```python
from build123d import *

# Parameters (mm, degrees)
SKETCH1_R           = 1.275
BOSS_EXTRUDE1_DEPTH = 6.5
SKETCH2_W           = 3.53
SKETCH2_H           = 1.96
BOSS_EXTRUDE2_DEPTH = 1.45
FILLET1_R           = 0.7
SKETCH3_W           = 3.2
SKETCH3_H           = 0.56
SKETCH3_H_2         = 0.5
BOSS_EXTRUDE3_DEPTH = 0.9
SKETCH4_W           = 1.2
SKETCH4_H           = 0.56
SKETCH4_H_2         = 0.5
BOSS_EXTRUDE4_DEPTH = 3.47
FILLET2_R           = 0.59


with BuildPart() as part:
    # Sketch1 → Boss-Extrude1 (new body)
    with BuildSketch(Plane(origin=(0, 0, 0), x_dir=(0, 0, -1), z_dir=(1, 0, 0))):
        with BuildLine():
            Line((-37.373122581, 0), (-34.673122581, 0))
            Line((-34.673122581, 0), (-34.673122581, -0.45))
            Line((-34.673122581, -0.45), (-30.873122581, -0.45))
            Line((-30.873122581, -0.45), (-30.873122581, 0))
            Line((-30.873122581, 0), (-24.973122581, 0))
            Line((-24.973122581, 0), (-24.973122581, -0.45))
            Line((-24.973122581, -0.45), (-21.173122581, -0.45))
            Line((-21.173122581, -0.45), (-21.173122581, 0))
            Line((-21.173122581, 0), (-18.673122581, 0))
            ThreePointArc((-18.673122581, 0), (-18.31956919, 0.146446609), (-18.173122581, 0.5))
            Line((-18.173122581, 0.5), (-18.173122581, 9.02))
            ThreePointArc((-18.173122581, 9.02), (-18.31956919, 9.373553391), (-18.673122581, 9.52))
            Line((-18.673122581, 9.52), (-28.173122581, 9.52))
            Line((-28.173122581, 9.52), (-28.173122581, 10.16))
            Line((-28.173122581, 10.16), (-37.373122581, 10.16))
            ThreePointArc((-37.373122581, 10.16), (-37.726675972, 10.013553391), (-37.873122581, 9.66))
            Line((-37.873122581, 9.66), (-37.873122581, 0.5))
            ThreePointArc((-37.873122581, 0.5), (-37.726675972, 0.146446609), (-37.373122581, 0))
        make_face()
        with Locations((-32.773122581, 2.525)):
            Circle(SKETCH1_R, mode=Mode.SUBTRACT)
        with Locations((-23.073122581, 2.525)):
            Circle(SKETCH1_R, mode=Mode.SUBTRACT)
    extrude(amount=BOSS_EXTRUDE1_DEPTH)

    # Sketch2 → Boss-Extrude2 (add)
    with BuildSketch(Plane(origin=(0, 10.16, 0), x_dir=(1, 0, 0), z_dir=(0, 1, 0))):
        with Locations((3.635, -30.693122581)):
            Rectangle(SKETCH2_W, SKETCH2_H)
    extrude(amount=BOSS_EXTRUDE2_DEPTH)

    # Fillet1
    fillet1_edges = [part.edges().sort_by_distance(p)[0] for p in [
        (3.635, 11.61, 31.673122581),
        (3.635, 11.61, 29.713122581),
    ]]
    fillet(fillet1_edges, radius=FILLET1_R)

    # Sketch3 → Boss-Extrude3 (add)
    with BuildSketch(Plane(origin=(0, 0, 0), x_dir=(-1, 0, 0), z_dir=(0, -1, 0))):
        with Locations((-3.25, -36.193122581)):
            Rectangle(SKETCH3_W, SKETCH3_H)
        with Locations((-3.25, -27.223122581)):
            Rectangle(SKETCH3_W, SKETCH3_H_2)
        with Locations((-3.25, -20.023122581)):
            Rectangle(SKETCH3_W, SKETCH3_H_2)
    extrude(amount=BOSS_EXTRUDE3_DEPTH)

    # Sketch4 → Boss-Extrude4 (add)
    with BuildSketch(Plane(origin=(0, -0.9, 0), x_dir=(-1, 0, 0), z_dir=(0, -1, 0))):
        with Locations((-3.25, -36.193122581)):
            Rectangle(SKETCH4_W, SKETCH4_H)
        with Locations((-3.25, -27.223122581)):
            Rectangle(SKETCH4_W, SKETCH4_H_2)
        with Locations((-3.25, -20.023122581)):
            Rectangle(SKETCH4_W, SKETCH4_H_2)
    extrude(amount=BOSS_EXTRUDE4_DEPTH)

    # Fillet2
    fillet2_edges = [part.edges().sort_by_distance(p)[0] for p in [
        (2.65, -4.37, 36.193122581),
        (3.85, -4.37, 36.193122581),
        (2.65, -4.37, 27.223122581),
        (3.85, -4.37, 27.223122581),
        (3.85, -4.37, 20.023122581),
        (2.65, -4.37, 20.023122581),
    ]]
    fillet(fillet2_edges, radius=FILLET2_R)


solid = part.part
```
Work out the finished part from the listing and answer in its coordinate system (mm). A direction names the side the tool comes from. Round coordinates to 2 decimals unless told otherwise and drop trailing zeros. Loops run counter-clockwise (first coordinate to the right, second up) from the corner with the lowest first, then second, coordinate; pieces in that order, holes last.
(1) The part is cut by section C-C, the plane x = 0.75. Give the vertices of the cut face in (y, z) (3 decimals).
Computed values:
outline: (-0.45, 21.173) - (0, 21.173) - (0, 18.673) arc R0.5 ccw to (0.5, 18.173) - (9.02, 18.173) arc R0.5 ccw to (9.52, 18.673) - (9.52, 28.173) - (10.16, 28.173) - (10.16, 37.373) arc R0.5 ccw to (9.66, 37.873) - (0.5, 37.873) arc R0.5 ccw to (0, 37.373) - (0, 34.673) - (-0.45, 34.673) - (-0.45, 30.873) - (0, 30.873) - (0, 24.973) - (-0.45, 24.973) - close; hole circle Ø2.55 at (2.525, 23.073); hole circle Ø2.55 at (2.525, 32.773)
(2) Each of these flat-tipped pins is pushed along its axis until it touches: P1, Ø1, axis at y = 4.5, z = 24, coming from the -X side; P2, Ø1.6, axis at x = 4, y = -3, coming from the -Z side; P3, Ø3.5, axis at x = 3, y = -1.5, coming from the +Z side; P4, Ø1.6, axis at y = 11, z = 30.5, coming from the +X side. Where does it stop, or does it pass through?
Computed values:
P1: stops at x = 0
P2: stops at z = 19.77
P3: stops at z = 37.81
P4: stops at x = 5.4
(3) The part is cut by section D-D, the plane y = 2.75. Give the vertices of the cut face in (x, z).
Computed values:
outline: (0, 18.17) - (6.5, 18.17) - (6.5, 21.82) - (0, 21.82) - close; (0, 24.33) - (6.5, 24.33) - (6.5, 31.52) - (0, 31.52) - close; (0, 34.03) - (6.5, 34.03) - (6.5, 37.87) - (0, 37.87) - close
(4) The mould has two halves that part along Y. Classify faces 1 (the flat face through (3, -2, 36.473)), 2 (the flat face through (3, -0.45, 23)), 3 (the cylindrical face through (3.204, 2.581, 24.347)): pulls with the +Y half, pulls with the -Y half, needs draft (parallel to the pull), parting line crosses it, or undercut.
Computed values:
face 1: needs draft
face 2: pulls with the -Y half
face 3: undercut
(5) The part is cut by section B-B, the plane z = 24. Give the vertices of the cut face in (x, y).
Computed values:
outline: (0, -0.45) - (6.5, -0.45) - (6.5, 1.65) - (0, 1.65) - close; (0, 3.4) - (6.5, 3.4) - (6.5, 9.52) - (0, 9.52) - close
(6) For faces 4 (the flat face through (3, -2, 19.773)), 5 (the flat face through (1.87, 11, 31)), 6 (the flat face through (3, -2, 35.913)), determine the directions among +Z, -Z, +X, -X, +Y, -Y from which every point of the face is accessible in a straight line to the end or side of a thin tool.
Computed values:
face 4: -Z, +X, -X, -Y
face 5: +Z, -Z, -X, +Y
face 6: +X, -X, -Y
(7) Find the intervals of material crossed by L1, parallel to Z at x = 2, y = 2.5; L2, parallel to Z at x = 3.75, y = -0.75; L3, parallel to Y at x = 3, z = 35.25, in increasing order.
Computed values:
L1: z = 18.17 to 21.8, 24.35 to 31.5, 34.05 to 37.87
L2: z = 19.77 to 20.27, 26.97 to 27.47, 35.91 to 36.47
L3: y = 0 to 10.16
(8) The part is cut by section A-A, the plane y = -2.5. Give the vertices of the cut face in (x, z).
Computed values:
outline: (2.65, 19.77) - (3.85, 19.77) - (3.85, 20.27) - (2.65, 20.27) - close; (2.65, 26.97) - (3.85, 26.97) - (3.85, 27.47) - (2.65, 27.47) - close; (2.65, 35.91) - (3.85, 35.91) - (3.85, 36.47) - (2.65, 36.47) - close
